Could you check a few things on this model? Use its own coordinates, in mm. A direction names the side the tool comes from. Coordinates: 2 decimals unless noted, no trailing zeros. Write each loop counter-clockwise with the first axis right and the second up, starting at its lowest first coordinate (ties: lowest second). Pieces come first, ordered by that corner, then holes.
```python
from build123d import *

# Parameters (mm, degrees)
SKETCH048_R  = 1.775161
PAD043_DEPTH = 2.5
PAD044_DEPTH = 2.5


with BuildPart() as right_assembly_insect_leg_chain:
    # Sketch048 → Pad043 (new body)
    with BuildSketch(Plane(origin=(21.5, 17, 18.5124), x_dir=(1, 0, 0), z_dir=(0, 0, 1))):
        with BuildLine():
            ThreePointArc((14.5613, 6.51014), (15.942406, 34.290704), (14.588209, 62.072593))
            ThreePointArc((20.466069, 62.072593), (17.527139, 64.772596), (14.588209, 62.072593))
            ThreePointArc((20.466069, 62.072593), (19.206566, 34.284518), (20.683621, 6.507156))
            ThreePointArc((14.5613, 6.51014), (17.620969, 3.448525), (20.683621, 6.507156))
        make_face()
        with Locations((17.527139, 61.823095)):
            Circle(SKETCH048_R, mode=Mode.SUBTRACT)
        with Locations((17.717781, 6.510143)):
            Circle(SKETCH048_R, mode=Mode.SUBTRACT)
    extrude(amount=PAD043_DEPTH)

    # Sketch060 → Pad044 (new body)
    with BuildSketch(Plane(origin=(21.5, 17, 21.0124), x_dir=(1, 0, 0), z_dir=(0, 0, 1))):
        with BuildLine():
            Line((20.000001, 59.398018), (18.351276, 59.398018))
            Line((18.351276, 59.398018), (16.30761, 56.651009))
            Line((16.30761, 56.651009), (16.30761, 42.307617))
            Line((16.30761, 42.307617), (16.30761, 26.311142))
            Line((16.30761, 26.311142), (16.30761, 16.418461))
            Line((16.30761, 16.418461), (18, 11.53899))
            ThreePointArc((21.743425, 8.667282), (20.323658, 10.692271), (18, 11.53899))
            ThreePointArc((21.743425, 8.667282), (21.321037, 11.586215), (19.626274, 14))
            Line((19.626274, 14), (17.339302, 20.540378))
            ThreePointArc((21.117151, 17.667282), (19.683694, 19.702728), (17.339302, 20.540378))
            ThreePointArc((21.117151, 17.667282), (20.694763, 20.586215), (19, 23))
            Line((19, 23), (16.999998, 32.601983))
            ThreePointArc((21, 29.601985), (19.494884, 31.761832), (16.999998, 32.601983))
            ThreePointArc((21, 29.601985), (20.620642, 32.530944), (19, 35))
            Line((19, 35), (17, 45.62257))
            ThreePointArc((21.338368, 42.601985), (19.698982, 44.873209), (17, 45.62257))
            ThreePointArc((21.338368, 42.601985), (20.95901, 45.530944), (19.338368, 48))
            Line((19.338368, 48), (18, 57.000001))
            ThreePointArc((22.000001, 54.000003), (20.494886, 56.159849), (18, 57.000001))
            ThreePointArc((22.000001, 54.000003), (21.620643, 56.928962), (20.000001, 59.398018))
        make_face()
    extrude(amount=-PAD044_DEPTH)


with BuildPart() as part_mirroring007:
    # Part__Mirroring007: instance of right_assembly_insect_leg_chain
    add(right_assembly_insect_leg_chain.part.mirror(Plane(origin=(0, 0, 0), x_dir=(0, -1, 0), z_dir=(1, 0, 0))))


with BuildPart() as part_mirroring007_1:
    # Part__Mirroring007 placement: moved
    add(part_mirroring007.part.moved(Location((0, 0.15, 0))))


solid = part_mirroring007_1.part
```
1. If we mould it in two halves opening along Y, with no side actions, what happens to faces 4 (the face through (-42.506, 62.55, 19.78)), 5 (the face through (-39, 52, 18.512)), 6 (the face through (-39.98, 80.47, 19.74))? For each: pulls with the +Y half, pulls with the -Y half, needs draft (parallel to the pull), parting line crosses it, or undercut.
Verdict:
face 4: undercut
face 5: needs draft
face 6: undercut
2. I want a section at A-A on x = -39. Please give me the cut outline in (y, z).
Verdict:
outline: (20.6, 18.51) - (21.9, 18.51) - (21.9, 21.01) - (20.6, 21.01) - close; (25.42, 18.51) - (77.2, 18.51) - (77.2, 21.01) - (25.42, 21.01) - close; (80.75, 18.51) - (81.92, 18.51) - (81.92, 21.01) - (80.75, 21.01) - close
3. For pin 1 (1.5 mm diameter, centred on x = -42.5, z = 20.5, fed in from +Y); pin 2 (1.5 mm diameter, centred on x = -41.5, z = 20.5, fed in from -Y), each with a flat end and sliding along its axis, tell me the tip position at first contact or that it passes through.
Verdict:
pin 1: stops at y = 80.11
pin 2: stops at y = 21.07
4. Please list where these lines run through material, in increasing order: line 1 along Y through (x, z) = (-40.25, 19.1); line 2 along Y through (x, z) = (-37.75, 18.9); line 3 along X through (y, z) = (72, 19.1).
Verdict:
line 1: y = 20.81 to 22.22, 25.1 to 77.69, 80.26 to 81.66
line 2: y = 20.92 to 22.66, 24.66 to 77.74, 80.21 to 81.63
line 3: x = -43.53 to -43.14, -41.37 to -36.7
5. On a 3-axis mill with a long thin cutter (end or side, diameter ignored), from which of +Z, -Z, +X, -X, +Y, -Y can I reach the whole of each face in a straight line? I mean faces 1 (the face through (-41.835, 77.802, 19.745)), 2 (the face through (-37.44, 51.05, 19.74)), 3 (the face through (-40.82, 44.44, 19.74)). Say none if no direction works.
Verdict:
face 1: +Z, -Z, -X
face 2: +Z, -Z, +X
face 3: +Z, -Z
6. I want a section at D-D on y = 45.5. Please give me the cut outline in (x, z).
Verdict:
outline: (-40.79, 18.51) - (-37.38, 18.51) - (-37.38, 21.01) - (-40.79, 21.01) - close
7. I want a section at B-B on z = 19.05. Please give me the cut outline in (x, y), plus the area to 3 significant figures.
Verdict:
outline: (-43.5, 71.15) arc R4.2 cw to (-41.49, 73.63) arc R282.75 cw to (-40.98, 65.01) arc R6.59 ccw to (-42.84, 59.75) arc R4.23 cw to (-40.87, 62.23) arc R282.75 cw to (-40.71, 51.94) arc R6.59 ccw to (-42.5, 46.75) arc R4.2 cw to (-40.73, 49.1) arc R282.75 cw to (-41, 39.66) arc R6.35 ccw to (-42.62, 34.82) arc R4.12 cw to (-41.14, 36.89) arc R282.75 cw to (-41.55, 30.74) arc R6.35 ccw to (-43.24, 25.82) arc R4.12 cw to (-41.78, 27.87) arc R282.75 cw to (-42.18, 23.66) arc R3.06 ccw to (-36.06, 23.66) arc R282.85 cw to (-36.09, 79.22) arc R2.95 ccw to (-41.97, 79.22) arc R282.75 cw to (-41.71, 76.34) arc R6.59 ccw to start; hole circle Ø3.55 at (-39.22, 23.66); hole circle Ø3.55 at (-39.03, 78.97)
area: 259 mm2
8. I want a section at C-C on y = 29. Please give me the cut outline in (x, z), plus the area to 3 significant figures.
Verdict:
outline: (-42.71, 18.51) - (-36.54, 18.51) - (-36.54, 21.01) - (-42.71, 21.01) - close
area: 15.4 mm2
